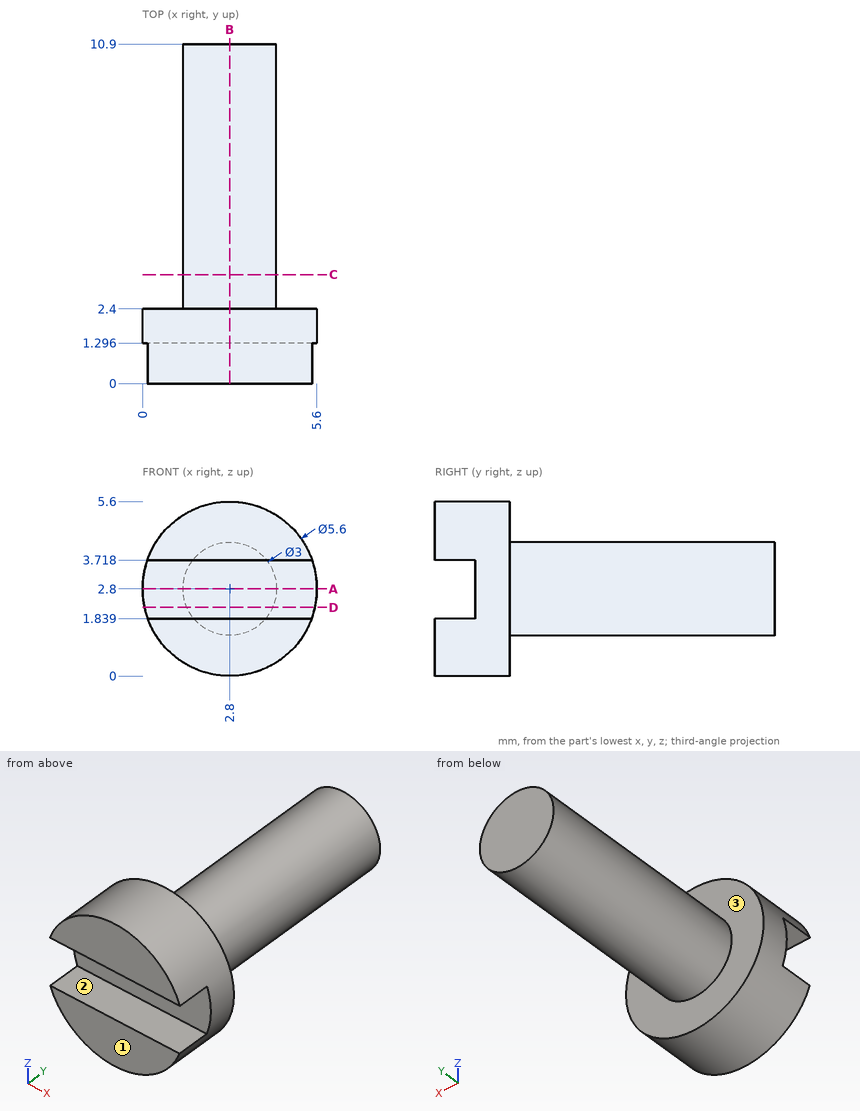
Print and shaded views of the part. All mm, measured from the part's lowest x, y and z. A direction names the side the tool comes from. Give positions to 0.01 mm unless a question says otherwise; leave off trailing zeros. Loops run counter-clockwise (first coordinate to the right, second up) from the corner with the lowest first, then second, coordinate; pieces in that order, holes last. Notation, with made-up numbers: (84.25, 21.5) -> (103.25, 21.5) arc R34 ccw to (103.25, 56.5) -> close; hole circle Ø1 at (45, -36). An arc over 180 degrees is marked (long way). Use a Markdown table: item, result.
1. Flat gauge pins, fed straight in: pin 1 (2 mm diameter, centred on y = 5.5, z = 5, fed in from +X); pin 2 (1.5 mm diameter, centred on x = 2, y = 6.5, fed in from -Z); pin 3 (1 mm diameter, centred on x = 1.5, y = 0.5, fed in from -Z). Where does each tip first touch, or does it go through?
Check result:
| item | result |
|---|---|
| pin 1 | stops at x = 3.7 |
| pin 2 | stops at z = 1.3 |
| pin 3 | stops at z = 0.12 |
2. Slice it at B-B (x = 2.8). List the corners of the cut face in (y, z).
Check result:
| item | result |
|---|---|
| outline | (0, 0) -> (2.4, 0) -> (2.4, 1.3) -> (10.9, 1.3) -> (10.9, 4.3) -> (2.4, 4.3) -> (2.4, 5.6) -> (0, 5.6) -> (0, 3.72) -> (1.3, 3.72) -> (1.3, 1.84) -> (0, 1.84) -> close |
3. Slice it at D-D (z = 2.2). List the corners of the cut face in (x, y) (1 decimal), plus the area to 3 significant figures.
Check result:
| item | result |
|---|---|
| outline | (0.1, 1.3) -> (5.5, 1.3) -> (5.5, 2.4) -> (4.2, 2.4) -> (4.2, 10.9) -> (1.4, 10.9) -> (1.4, 2.4) -> (0.1, 2.4) -> close |
| area | 29.4 mm^2 |
4. Wall check: L1, parallel to Y at x = 4, z = 4.8; L2, parallel to Y at x = 5.2, z = 2.6; L3, parallel to Z at x = 0.35, y = 1 (1 decimal). Give the ranges that are in metal, low to high. Write a range as [from, to].
Check result:
| item | result |
|---|---|
| L1 | y = [0, 2.4] |
| L2 | y = [1.3, 2.4] |
| L3 | z = [1.4, 1.8], [3.7, 4.2] |
5. Which spindle directions (+Z, -Z, +X, -X, +Y, -Y) get a long thin tool onto all of the face, cutting with end or side? Do the marked faces 1, 2 and 3. Say none if no direction does.
Check result:
| item | result |
|---|---|
| face 1 | +Z, -Z, +X, -X, -Y |
| face 2 | +X, -X, -Y |
| face 3 | +Y |
6. Slice it at A-A (z = 2.8). List the corners of the cut face in (x, y).
Check result:
| item | result |
|---|---|
| outline | (0, 1.3) -> (5.6, 1.3) -> (5.6, 2.4) -> (4.3, 2.4) -> (4.3, 10.9) -> (1.3, 10.9) -> (1.3, 2.4) -> (0, 2.4) -> close |
7. Slice it at C-C (y = 3.5). List the corners of the cut face in (x, z).
Check result:
| item | result |
|---|---|
| outline | circle Ø3 at (2.8, 2.8) |
